Check sheet for the modelled part. Datum: model origin and axes. Units: mm. A direction names the side the tool comes from. Coordinates: 2 decimals unless noted, no trailing zeros. Loops run counter-clockwise (first coordinate to the right, second up) from the corner with the lowest first, then second, coordinate; pieces in that order, holes last. Notation, with made-up numbers: M -14.75,-2.5 L 33.25,-2.5 A19 ccw 33.25,33.5 Z; hole C 24.25,-9 d10. An arc over 180 degrees is marked long. Answer in a Markdown table with one row per item. Add a question column.
```python
from build123d import *

# Parameters (mm, degrees)
SKETCH1_W               = 45.2
SKETCH1_H               = 21
BOSS_EXTRUDE1_DEPTH     = 0.75
SKETCH2_R               = 1
CUT_EXTRUDE1_DEPTH      = 2.5
MIRROR2_COPY_1_SKETCH_R = 1
MIRROR2_COPY_1_DEPTH    = 2.5
SKETCH3_R               = 8
BOSS_EXTRUDE2_DEPTH     = 10
SKETCH9_R               = 7.25
CUT_EXTRUDE2_DEPTH      = 8
FILLET1_R               = 0.3
SKETCH10_R              = 5.6
BOSS_EXTRUDE3_DEPTH     = 4


with BuildPart() as part:
    # Sketch1 → Boss-Extrude1 (new body, symmetric)
    with BuildSketch(Plane.XY):
        Rectangle(SKETCH1_W, SKETCH1_H)
    extrude(amount=BOSS_EXTRUDE1_DEPTH, both=True)

    # Sketch2 → Cut-Extrude1 (cut, through all)
    with BuildSketch(Plane.XY.offset(0.75)):
        with Locations((-18.596547757, 7.099196252)):
            Circle(SKETCH2_R)
    cut_extrude1 = extrude(amount=-CUT_EXTRUDE1_DEPTH, mode=Mode.SUBTRACT)

    # Mirror1: Cut-Extrude1 across plane
    add(cut_extrude1.mirror(Plane(origin=(0, 0, 0), x_dir=(0, 0, 1), z_dir=(1, 0, 0))), mode=Mode.SUBTRACT)

    # Mirror2: Cut-Extrude1 across plane
    add(cut_extrude1.mirror(Plane.ZX), mode=Mode.SUBTRACT)

    # Mirror2 copy 1 sketch → Mirror2 copy 1 (cut, through all)
    with BuildSketch(Plane(origin=(0, 0, 0.75), x_dir=(-1, 0, 0), z_dir=(0, 0, 1))):
        with Locations((-18.596547757, 7.099196252)):
            Circle(MIRROR2_COPY_1_SKETCH_R)
    extrude(amount=-MIRROR2_COPY_1_DEPTH, mode=Mode.SUBTRACT)

    # Sketch3 → Boss-Extrude2 (add)
    with BuildSketch(Plane.XY.offset(0.75)):
        with Locations((-11, 0)):
            Circle(SKETCH3_R)
    boss_extrude2 = extrude(amount=BOSS_EXTRUDE2_DEPTH)

    # Sketch9 → Cut-Extrude2 (cut)
    with BuildSketch(Plane.XY.offset(10.75)):
        with Locations((-11, 0)):
            Circle(SKETCH9_R)
    cut_extrude2 = extrude(amount=-CUT_EXTRUDE2_DEPTH, mode=Mode.SUBTRACT)

    # Mirror3: Boss-Extrude2 across plane
    add(boss_extrude2.mirror(Plane(origin=(0, 0, 0), x_dir=(0, 0, 1), z_dir=(1, 0, 0))))

    # Mirror4: Cut-Extrude2 across plane
    add(cut_extrude2.mirror(Plane(origin=(0, 0, 0), x_dir=(0, 0, 1), z_dir=(1, 0, 0))), mode=Mode.SUBTRACT)

    # Fillet1
    fillet1_edges = [part.edges().sort_by_distance(p)[0] for p in [
        (-19, 0, 0.75),
        (-19, 0, 10.75),
        (19, 0, 0.75),
        (19, 0, 10.75),
    ]]
    fillet(fillet1_edges, radius=FILLET1_R)

    # Sketch10 → Boss-Extrude3 (add)
    with BuildSketch(Plane.XY.offset(2.75)):
        with Locations((-11, 0)):
            Circle(SKETCH10_R)
    boss_extrude3 = extrude(amount=BOSS_EXTRUDE3_DEPTH)

    # Mirror5: Boss-Extrude3 across plane
    add(boss_extrude3.mirror(Plane(origin=(0, 0, 0), x_dir=(0, 0, 1), z_dir=(1, 0, 0))))


solid = part.part
```
Q1. Thickness scan on L1, parallel to Y at x = -11, z = 7.5; L2, parallel to X at y = 1.5, z = 5.5; L3, parallel to Z at x = -10, y = 8.75. Record the ranges inside material, lowest first.
Q2. Cross-section at C-C (x = 11). Record the cut outline in (y, z), plus the area to 3 significant figures.
Q3. Cross-section at B-B (z = 8.75). Record the cut outline in (x, y), plus the area to 3 significant figures.
Q4. Mould release check, pull along Y, two halves, no side actions. Record for faces 1 (the face through (0, 0, -0.75)), 2 (the face through (0, 10.5, 0)), 3 (the face through (4.303, -2.777, 6.806)): released by +Y, released by -Y, zero draft, split by the parting line, or undercut.
Q5. Cross-section at A-A (z = 5.25). Record the cut outline in (x, y).
Q6. Go/stop test with flat-tipped pins: pin 1 (6 mm diameter, centred on x = 12.5, y = -1.5, fed in from +Z); pin 2 (6 mm diameter, centred on x = -1, y = -7, fed in from +Z); pin 3 (2 mm diameter, centred on y = 4, z = 4.5, fed in from -X). Record where each tip stops, or that it passes through.
Q7. Access from +Z, -Z, +X, -X, +Y, -Y to the whole of each face (thin tool, end or side, straight path). Record for faces 4 (the face through (-8, -5, 2.75)), 5 (the face through (0, -10.5, 0)).
Q8. Cross-section at D-D (y = -8.75). Record the cut outline in (x, z), plus the area to 3 significant figures.
Answer key:
| question | item | result |
|---|---|---|
| 1 | L1 | -8 to -7.25, 7.25 to 8 |
| 1 | L2 | -18.86 to -18.09, -16.4 to -5.6, -3.91 to -3.14, 3.14 to 3.91, 5.6 to 16.4, 18.09 to 18.86 |
| 1 | L3 | -0.75 to 0.75 |
| 2 | outline | M -10.5,-0.75 L 10.5,-0.75 L 10.5,0.75 L 8.3,0.75 A0.3 cw 8,1.05 L 8,10.45 A0.3 ccw 7.7,10.75 L 7.25,10.75 L 7.25,2.75 L 5.6,2.75 L 5.6,6.75 L -5.6,6.75 L -5.6,2.75 L -7.25,2.75 L -7.25,10.75 L -7.7,10.75 A0.3 ccw -8,10.45 L -8,1.05 A0.3 cw -8.3,0.75 L -10.5,0.75 Z |
| 2 | area | 120 mm^2 |
| 3 | outline | C -11,0 d16; C 11,0 d16; hole C -11,0 d14.5; hole C 11,0 d14.5 |
| 3 | area | 71.9 mm^2 |
| 4 | face 1 | zero draft |
| 4 | face 2 | released by +Y |
| 4 | face 3 | undercut |
| 5 | outline | C -11,0 d16; C -11,0 d11.2; C 11,0 d16; C 11,0 d11.2; hole C -11,0 d14.5; hole C 11,0 d14.5 |
| 6 | pin 1 | z = 6.75 |
| 6 | pin 2 | z = 0.75 |
| 6 | pin 3 | x = -18.42 |
| 7 | face 4 | +Z |
| 7 | face 5 | +Z, -Z, +X, -X, -Y |
| 8 | outline | M -22.6,-0.75 L 22.6,-0.75 L 22.6,0.75 L -22.6,0.75 Z |
| 8 | area | 67.8 mm^2 |
